Design review of the part built by this model. Coordinates are the model's own, in mm. Face numbers are marked on the shaded views. A direction names the side the tool comes from. Coordinates: 2 decimals unless noted, no trailing zeros. Loops run counter-clockwise (first coordinate to the right, second up) from the corner with the lowest first, then second, coordinate; pieces in that order, holes last. Notation, with made-up numbers: (44.25, 18) - (75.25, 18) arc R6 cw to (75.25, 24) - close; hole circle Ø8 at (-29.75, 65.25). An arc over 180 degrees is marked (long way). One line per question, with ' | ' between items.
from build123d import *

# Parameters (mm, degrees)
BOSS_EXTRUDE1_DEPTH = 20


with BuildPart() as part:
    # Sketch1 → Boss-Extrude1 (new body)
    with BuildSketch(Plane.XY):
        with BuildLine():
            Line((22, 0), (-22, 0))
            Line((-22, 0), (-22, -18))
            ThreePointArc((-22, -18), (-22.585786438, -19.414213562), (-24, -20))
            Line((-24, -20), (-40, -20))
            ThreePointArc((-40, -20), (-41.414213562, -19.414213562), (-42, -18))
            Line((-42, -18), (-42, -10))
            ThreePointArc((-42, -10), (-44.928932188, -2.928932188), (-52, 0))
            Line((-52, 0), (-75, 0))
            ThreePointArc((-75, 0), (-76.414213562, 0.585786438), (-77, 2))
            Line((-77, 2), (-77, 10.857864376))
            ThreePointArc((-77, 10.857864376), (-76.238795325, 14.6846987), (-74.071067812, 17.928932188))
            Line((-74.071067812, 17.928932188), (-61.928932188, 30.071067812))
            ThreePointArc((-61.928932188, 30.071067812), (-58.6846987, 32.238795325), (-54.857864376, 33))
            Line((-54.857864376, 33), (54.857864376, 33))
            ThreePointArc((54.857864376, 33), (58.6846987, 32.238795325), (61.928932188, 30.071067812))
            Line((61.928932188, 30.071067812), (74.071067812, 17.928932188))
            ThreePointArc((74.071067812, 17.928932188), (76.238795325, 14.6846987), (77, 10.857864376))
            Line((77, 10.857864376), (77, 2))
            ThreePointArc((77, 2), (76.414213562, 0.585786438), (75, 0))
            Line((75, 0), (52, 0))
            ThreePointArc((52, 0), (44.928932188, -2.928932188), (42, -10))
            Line((42, -10), (42, -18))
            ThreePointArc((42, -18), (41.414213562, -19.414213562), (40, -20))
            Line((40, -20), (24, -20))
            ThreePointArc((24, -20), (22.585786438, -19.414213562), (22, -18))
            Line((22, -18), (22, 0))
        make_face()
    extrude(amount=BOSS_EXTRUDE1_DEPTH)


solid = part.part
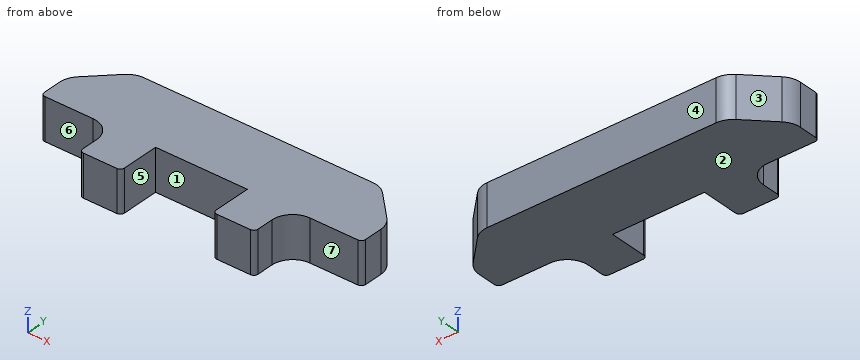
Q1. Take a section at A-A (y = -15). Give the boundary of the cut face in (x, z), plus the area to 3 significant figures.
Returned:
outline: (-42, 0) - (-22, 0) - (-22, 20) - (-42, 20) - close; (22, 0) - (42, 0) - (42, 20) - (22, 20) - close | area: 800 mm²
Q2. Take a section at B-B (z = 4). Give the boundary of the cut face in (x, y).
Returned:
outline: (-77, 2) arc R2 ccw to (-75, 0) - (-52, 0) arc R10 cw to (-42, -10) - (-42, -18) arc R2 ccw to (-40, -20) - (-24, -20) arc R2 ccw to (-22, -18) - (-22, 0) - (22, 0) - (22, -18) arc R2 ccw to (24, -20) - (40, -20) arc R2 ccw to (42, -18) - (42, -10) arc R10 cw to (52, 0) - (75, 0) arc R2 ccw to (77, 2) - (77, 10.86) arc R10 ccw to (74.07, 17.93) - (61.93, 30.07) arc R10 ccw to (54.86, 33) - (-54.86, 33) arc R10 ccw to (-61.93, 30.07) - (-74.07, 17.93) arc R10 ccw to (-77, 10.86) - close
Q3. To check wall thickness, follow line 1 along X through (y, z) = (-15, 4.25); line 2 along Y through (x, z) = (-11, 3); line 3 along X through (y, z) = (-1.5, 3). State the ranges of each line that lie inside material, in increasing order.
Returned:
line 1: x = -42 to -22, 22 to 42 | line 2: y = 0 to 33 | line 3: x = -46.73 to -22, 22 to 46.73
Q4. Tool access review of the marked faces 4, 5, 6 and 7: name each direction out of +Z, -Z, +X, -X, +Y, -Y from which nothing blocks a thin tool from reaching the whole face with its end or side.
Returned:
face 4: +Z, -Z, +X, -X, +Y | face 5: +Z, -Z, -Y | face 6: +Z, -Z, -X, -Y | face 7: +Z, -Z, +X, -Y
Q5. For pin 1 (9 mm diameter, centred on y = -12, z = 14.5, fed in from -X); pin 2 (12 mm diameter, centred on y = -13.5, z = 15.5, fed in from +X); pin 3 (5.5 mm diameter, centred on y = -7.5, z = 14, fed in from -X); pin 4 (4 mm diameter, centred on x = -42.5, y = 22, fed in from -Z), all flat-tipped, find the tip position at first contact; note any pin that passes through.
Returned:
pin 1: stops at x = -42.32 | pin 2: stops at x = 42.32 | pin 3: stops at x = -43.49 | pin 4: stops at z = 0
Q6. Draft analysis for pull direction X (two halves, no side actions). For the marked faces 1, 2 and 3, state which applies: +X half, -X half, draft (parallel to the pull), parting line (faces both ways), or undercut.
Returned:
face 1: undercut | face 2: draft | face 3: -X half
Q7. Take a section at D-D (y = 23). Give the boundary of the cut face in (x, z), plus the area to 3 significant figures.
Returned:
outline: (-69, 0) - (69, 0) - (69, 20) - (-69, 20) - close | area: 2,760 mm²
Q8. Take a section at C-C (x = 10.5). Give the boundary of the cut face in (y, z).
Returned:
outline: (0, 0) - (33, 0) - (33, 20) - (0, 20) - close
